```python
from build123d import *

# Parameters (mm, degrees)
KEYEDBODY_DEPTH  = 17
SKETCH2_R        = 4.1
SMALLSHAFT_DEPTH = 5


with BuildPart() as part:
    # Sketch1 → KeyedBody (new body)
    with BuildSketch(Plane.ZY.offset(18)):
        with BuildLine():
            Line((-3.441775952, 9.17573857), (-4.337445486, 11.509037479))
            ThreePointArc((-4.337445486, 11.509037479), (-7.229313618, 9.950296561), (-9.605400723, 7.681643964))
            Line((-9.605400723, 7.681643964), (-7.663078698, 6.108782601))
            ThreePointArc((-7.663078698, 6.108782601), (-9.32035386, 3.028366545), (-9.790213218, -0.437864293))
            Line((-9.790213218, -0.437864293), (-12.286089458, -0.568667624))
            ThreePointArc((-12.286089458, -0.568667624), (-11.697275149, -3.800675088), (-10.273909609, -6.76152042))
            Line((-10.273909609, -6.76152042), (-8.177819046, -5.400303292))
            ThreePointArc((-8.177819046, -5.400303292), (-5.760295472, -7.928366545), (-2.608908574, -9.446353585))
            Line((-2.608908574, -9.446353585), (-3.255775388, -11.860493399))
            ThreePointArc((-3.255775388, -11.860493399), (0, -12.299242946), (3.255775388, -11.860493399))
            Line((3.255775388, -11.860493399), (2.608908574, -9.446353585))
            ThreePointArc((2.608908574, -9.446353585), (5.760295472, -7.928366545), (8.177819046, -5.400303292))
            Line((8.177819046, -5.400303292), (10.273909609, -6.76152042))
            ThreePointArc((10.273909609, -6.76152042), (11.697275149, -3.800675088), (12.286089458, -0.568667624))
            Line((12.286089458, -0.568667624), (9.790213218, -0.437864293))
            ThreePointArc((9.790213218, -0.437864293), (9.32035386, 3.028366545), (7.663078698, 6.108782601))
            Line((7.663078698, 6.108782601), (9.605400723, 7.681643964))
            ThreePointArc((9.605400723, 7.681643964), (7.229313618, 9.950296561), (4.337445486, 11.509037479))
            Line((4.337445486, 11.509037479), (3.441775952, 9.17573857))
            ThreePointArc((3.441775952, 9.17573857), (0, 9.8), (-3.441775952, 9.17573857))
        make_face()
    extrude(amount=KEYEDBODY_DEPTH)

    # Sketch2 → SmallShaft (add)
    with BuildSketch(Plane.ZY.offset(35)):
        Circle(SKETCH2_R)
    extrude(amount=SMALLSHAFT_DEPTH)


solid = part.part
```
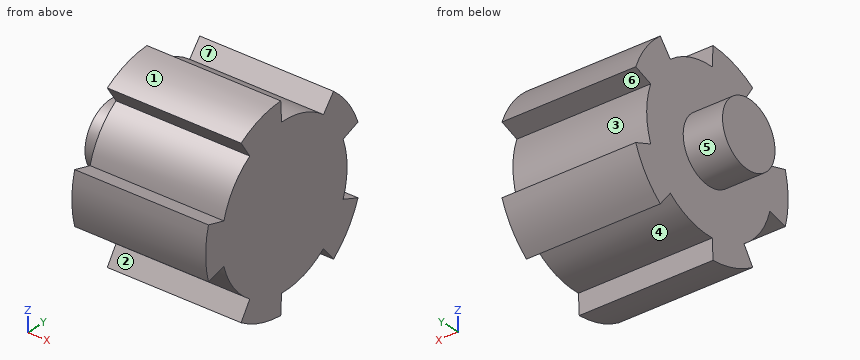
Geometry: final body of the model. Coordinates: model frame, mm. Face numbers are marked on the shaded views. A direction names the side the tool comes from. Round coordinates to 2 decimals unless told otherwise and drop trailing zeros. Order: outer loops, then holes, each group sorted by start corner. A loop starts at its lowest first (then second) coordinate and runs counter-clockwise, first axis right, second up. Notation, with made-up numbers: (-6.75, -39) -> (6.25, -39) arc R32 cw to (6.25, -9) -> close; hole circle Ø2 at (62.5, 27). An arc over 180 degrees is marked (long way). Use one line per item in the form item = value.
(1) Ray query, probe 1 along Z at (x, y) = (-28.5, -6.25); probe 2 along Y at (x, z) = (-25, 0.25); probe 3 along X at (y, z) = (-3, -8). Return the intervals inside material, ascending. Write a range as [from, to].
Results list:
probe_1 = [-10.59, -9.49], [-7.55, 7.55], [9.49, 10.59]
probe_2 = [-12.3, 9.8]
probe_3 = [-35, -18]
(2) First-contact query: pin 1 Ø6 at (x, z) = (-33, 9) entering from -Y; pin 2 Ø10 at (y, z) = (-10, 7.5) entering from -X; pin 3 Ø12 at (x, y) = (-23.5, -0.5) entering from -Z; pin 4 Ø6 at (x, z) = (-34.5, -5.5) entering from -Y. Flat tips, straight axial feed; report the tip coordinate or a pass-through.
Results list:
pin_1 = -7.75
pin_2 = -35
pin_3 = -12.29
pin_4 = -12.04
(3) Section A-A on y = 0. Return loops of the section in (x, z).
Results list:
outline = (-40, -4.1) -> (-35, -4.1) -> (-35, -9.8) -> (-18, -9.8) -> (-18, 9.8) -> (-35, 9.8) -> (-35, 4.1) -> (-40, 4.1) -> close
(4) Section D-D on x = -36. Return loops of the section in (y, z), and give its area (3 significant figures).
Results list:
outline = circle Ø8.2 at (0, 0)
area = 52.8 mm^2
(5) Draft query along Z for the marked faces 1, 2, 3 and 4. Return one class per face: pulls with the +Z half, pulls with the -Z half, needs draft (parallel to the pull), parting line crosses it, or undercut.
Results list:
face_1 = pulls with the +Z half
face_2 = undercut
face_3 = undercut
face_4 = pulls with the -Z half
(6) Section B-B on z = 0. Return loops of the section in (x, y).
Results list:
outline = (-40, -4.1) -> (-35, -4.1) -> (-35, -12.3) -> (-18, -12.3) -> (-18, 9.8) -> (-35, 9.8) -> (-35, 4.1) -> (-40, 4.1) -> close
(7) Access query for the marked faces 5, 6 and 7. Directions: +Z, -Z, +X, -X, +Y, -Y. A direction counts if a zero-diameter tool reaches every point of the face in a straight line with its end or side. Return the directions, or none.
Results list:
face_5 = -X
face_6 = +X, -X, +Y
face_7 = +Z, +X, -X
(8) Section C-C on x = -26.25. Return loops of the section in (y, z).
Results list:
outline = (-11.86, -3.26) -> (-9.45, -2.61) arc R9.8 ccw to (-5.4, -8.18) -> (-6.76, -10.27) arc R12.3 ccw to (-0.57, -12.29) -> (-0.44, -9.79) arc R9.8 ccw to (6.11, -7.66) -> (7.68, -9.61) arc R12.3 ccw to (11.51, -4.34) -> (9.18, -3.44) arc R9.8 ccw to (9.18, 3.44) -> (11.51, 4.34) arc R12.3 ccw to (7.68, 9.61) -> (6.11, 7.66) arc R9.8 ccw to (-0.44, 9.79) -> (-0.57, 12.29) arc R12.3 ccw to (-6.76, 10.27) -> (-5.4, 8.18) arc R9.8 ccw to (-9.45, 2.61) -> (-11.86, 3.26) arc R12.3 ccw to start
